Can you work these out from the model? Positions are in its coordinate system, mm. Give positions to 0.01 mm unless a question says otherwise; leave off trailing zeros. Loops run counter-clockwise (first coordinate to the right, second up) from the corner with the lowest first, then second, coordinate; pieces in that order, holes last. Notation, with made-up numbers: M -3.75,26.5 L 48.25,26.5 A22 cw 48.25,57.5 Z; hole C 23.25,-1.5 d9. An arc over 180 degrees is marked long. Use CSV: the item, a comma, the result in double quotes.
from build123d import *

# Parameters (mm, degrees)
SKETCH1_W           = 300
SKETCH1_H           = 50
SKETCH1_R           = 4
MAIN_DEPTH          = 10
SKETCH4_R           = 2.5
MOUNT_DEPTH         = 11
SKETCH3_R           = 1.85
BEARING_MOUNT_DEPTH = 11


with BuildPart() as part:
    # Sketch1 → main (new body)
    with BuildSketch(Plane(origin=(0, 0, 0), x_dir=(1, 0, 0), z_dir=(0, 1, 0))):
        with Locations((0, -5)):
            Rectangle(SKETCH1_W, SKETCH1_H)
        with Locations((-100, 0)):
            Circle(SKETCH1_R, mode=Mode.SUBTRACT)
        with Locations((100, 0)):
            Circle(SKETCH1_R, mode=Mode.SUBTRACT)
    extrude(amount=MAIN_DEPTH)

    # Sketch4 → mount (cut, through all)
    with BuildSketch(Plane(origin=(0, 10, 0), x_dir=(1, 0, 0), z_dir=(0, 1, 0))):
        with Locations((-140, 5)):
            Circle(SKETCH4_R)
        with Locations((-140, -15)):
            Circle(SKETCH4_R)
        with Locations((140, -15)):
            Circle(SKETCH4_R)
        with Locations((140, 5)):
            Circle(SKETCH4_R)
    extrude(amount=-MOUNT_DEPTH, mode=Mode.SUBTRACT)

    # Sketch3 → bearing_mount (cut, through all)
    with BuildSketch(Plane(origin=(0, 10, 0), x_dir=(1, 0, 0), z_dir=(0, 1, 0))):
        with Locations((-17.5, 8)):
            Circle(SKETCH3_R)
        with Locations((17.5, 8)):
            Circle(SKETCH3_R)
        with Locations((-17.5, -10)):
            Circle(SKETCH3_R)
        with Locations((17.5, -10)):
            Circle(SKETCH3_R)
    extrude(amount=-BEARING_MOUNT_DEPTH, mode=Mode.SUBTRACT)


solid = part.part
Q1. I'm going to push a flat-ended pin straight in: P1, Ø5, axis at x = -108, z = 2.5, coming from the -Y side. Where does the tip first touch, or does it pass through?
Model answer:
P1,"y = 0"
Q2. I want a section at A-A, the plane x = -100. Please give me the cut outline in (y, z), then the cut area to 3 significant figures.
Model answer:
outline,"M 0,-20 L 10,-20 L 10,-4 L 0,-4 Z; M 0,4 L 10,4 L 10,30 L 0,30 Z"
area,"420 mm2"
Q3. Please list where these lines run through material, in increasing order: L1, parallel to Z at x = 140, y = 2.5; L2, parallel to X at y = 3.5, z = 15; L3, parallel to Z at x = 17.5, y = 5.75. Write a range as from..to.
Model answer:
L1,"-20..-7.5, -2.5..12.5, 17.5..30"
L2,"-150..-142.5, -137.5..137.5, 142.5..150"
L3,"-20..-9.85, -6.15..8.15, 11.85..30"
Q4. If we mould it in two halves opening along Z, with no side actions, what happens to faces 1 (the flat face through (-2, 5, 30)), 2 (the cylindrical face through (103.695, 4.93, 1.532)), 3 (the flat face through (-2, 0, 5))? For each: released by +Z, released by -Z, zero draft, split by the parting line, or undercut.
Model answer:
face 1,"released by +Z"
face 2,"undercut"
face 3,"zero draft"
